Can you work these out from the model? Positions are in its coordinate system, mm. A direction names the side the tool comes from. Round coordinates to 2 decimals unless told otherwise and drop trailing zeros. Loops run counter-clockwise (first coordinate to the right, second up) from the corner with the lowest first, then second, coordinate; pieces in that order, holes last.
from build123d import *

# Parameters (mm, degrees)
SKETCH1_W           = 80
SKETCH1_H           = 160
SKETCH1_R           = 1.25
SKETCH1_R_2         = 1.5
SKETCH1_R_3         = 3.175
SKETCH1_W_2         = 25
SKETCH1_H_2         = 10
BOSS_EXTRUDE1_DEPTH = 3
SKETCH2_W           = 5
SKETCH2_H           = 25
BOSS_EXTRUDE2_DEPTH = 14
FILLET1_R           = 1
FILLET2_R           = 3
FILLET3_R           = 3
SKETCH4_R           = 1.25
CUT_EXTRUDE1_DEPTH  = 180.691402132
SKETCH6_R           = 2
CUT_EXTRUDE2_DEPTH  = 8.89
LPATTERN1_COUNT     = 6
LPATTERN1_PITCH     = 10
FILLET4_R           = 2


with BuildPart() as part:
    # Sketch1 → Boss-Extrude1 (new body)
    with BuildSketch(Plane(origin=(0, 0, 0), x_dir=(1, 0, 0), z_dir=(0, 1, 0))):
        with Locations((40, 80)):
            Rectangle(SKETCH1_W, SKETCH1_H)
        with Locations(Location((8, 130, 0), (0, 0, 270))):
            Circle(SKETCH1_R, mode=Mode.SUBTRACT)
        with Locations(Location((16, 130, 0), (0, 0, 270))):
            Circle(SKETCH1_R, mode=Mode.SUBTRACT)
        with Locations(Location((24, 130, 0), (0, 0, 270))):
            Circle(SKETCH1_R, mode=Mode.SUBTRACT)
        with Locations(Location((24, 122, 0), (0, 0, 270))):
            Circle(SKETCH1_R, mode=Mode.SUBTRACT)
        with Locations(Location((24, 114, 0), (0, 0, 270))):
            Circle(SKETCH1_R, mode=Mode.SUBTRACT)
        with Locations(Location((16, 114, 0), (0, 0, 270))):
            Circle(SKETCH1_R, mode=Mode.SUBTRACT)
        with Locations(Location((8, 114, 0), (0, 0, 270))):
            Circle(SKETCH1_R, mode=Mode.SUBTRACT)
        with Locations(Location((8, 122, 0), (0, 0, 270))):
            Circle(SKETCH1_R, mode=Mode.SUBTRACT)
        with Locations(Location((72, 130, 0), (0, 0, 90))):
            Circle(SKETCH1_R, mode=Mode.SUBTRACT)
        with Locations(Location((72, 122, 0), (0, 0, 90))):
            Circle(SKETCH1_R, mode=Mode.SUBTRACT)
        with Locations(Location((72, 114, 0), (0, 0, 90))):
            Circle(SKETCH1_R, mode=Mode.SUBTRACT)
        with Locations(Location((64, 114, 0), (0, 0, 90))):
            Circle(SKETCH1_R, mode=Mode.SUBTRACT)
        with Locations(Location((64, 130, 0), (0, 0, 90))):
            Circle(SKETCH1_R, mode=Mode.SUBTRACT)
        with Locations(Location((56, 130, 0), (0, 0, 90))):
            Circle(SKETCH1_R, mode=Mode.SUBTRACT)
        with Locations(Location((56, 122, 0), (0, 0, 90))):
            Circle(SKETCH1_R, mode=Mode.SUBTRACT)
        with Locations(Location((56, 114, 0), (0, 0, 90))):
            Circle(SKETCH1_R, mode=Mode.SUBTRACT)
        with Locations(Location((40, 17, 0), (0, 0, 270))):
            Circle(SKETCH1_R_2, mode=Mode.SUBTRACT)
        with Locations(Location((40, 74.5, 0), (0, 0, 270))):
            Circle(SKETCH1_R_2, mode=Mode.SUBTRACT)
        with Locations(Location((7, 7, 0), (0, 0, 270))):
            Circle(SKETCH1_R_3, mode=Mode.SUBTRACT)
        with Locations(Location((73, 7, 0), (0, 0, 90))):
            Circle(SKETCH1_R_3, mode=Mode.SUBTRACT)
        with Locations((40, 100)):
            Rectangle(SKETCH1_W_2, SKETCH1_H_2, mode=Mode.SUBTRACT)
    extrude(amount=BOSS_EXTRUDE1_DEPTH)

    # Sketch2 → Boss-Extrude2 (add)
    with BuildSketch(Plane(origin=(0, 3, 0), x_dir=(1, 0, 0), z_dir=(0, 1, 0))):
        with Locations((2.5, 27.5)):
            Rectangle(SKETCH2_W, SKETCH2_H)
        with Locations((77.5, 27.5)):
            Rectangle(SKETCH2_W, SKETCH2_H)
    extrude(amount=BOSS_EXTRUDE2_DEPTH)

    # Fillet1
    fillet1_edges = [part.edges().sort_by_distance(p)[0] for p in [
        (77.5, 3, -15),
        (75, 3, -27.5),
        (77.5, 3, -40),
        (2.5, 3, -40),
        (5, 3, -27.5),
        (2.5, 3, -15),
    ]]
    fillet(fillet1_edges, radius=FILLET1_R)

    # Fillet2
    fillet2_edges = [part.edges().sort_by_distance(p)[0] for p in [
        (0, 1.5, -160),
        (80, 1.5, -160),
        (80, 1.5, 0),
        (0, 1.5, 0),
    ]]
    fillet(fillet2_edges, radius=FILLET2_R)

    # Fillet3
    fillet3_edges = [part.edges().sort_by_distance(p)[0] for p in [
        (77.5, 17, -40),
        (77.5, 17, -15),
        (2.5, 17, -15),
        (2.5, 17, -40),
    ]]
    fillet(fillet3_edges, radius=FILLET3_R)

    # Sketch4 → Cut-Extrude1 (cut, through all)
    with BuildSketch(Plane.ZY):
        with Locations((-27.5, 8)):
            Circle(SKETCH4_R)
        with Locations((-35.5, 13)):
            Circle(SKETCH4_R)
        with Locations(Location((-19.5, 13, 0), (0, 0, 180))):
            Circle(SKETCH4_R)
    extrude(amount=-CUT_EXTRUDE1_DEPTH, mode=Mode.SUBTRACT)

    # Sketch6 → Cut-Extrude2 (cut)
    with BuildSketch(Plane(origin=(0, 3, 0), x_dir=(1, 0, 0), z_dir=(0, 1, 0))):
        with Locations(Location((6, 99.467444438, 0), (0, 0, 270))):
            Circle(SKETCH6_R)
        with Locations(Location((74, 99.467444438, 0), (0, 0, 270))):
            Circle(SKETCH6_R)
    cut_extrude2 = extrude(amount=-CUT_EXTRUDE2_DEPTH, mode=Mode.SUBTRACT)

    # LPattern1: Cut-Extrude2 ×6
    with Locations(*[(0, 0, i * LPATTERN1_PITCH) for i in range(1, LPATTERN1_COUNT)]):
        add(cut_extrude2, mode=Mode.SUBTRACT)

    # Fillet4
    fillet4_edges = [part.edges().sort_by_distance(p)[0] for p in [
        (52.5, 1.5, -95),
        (52.5, 1.5, -105),
        (27.5, 1.5, -105),
        (27.5, 1.5, -95),
    ]]
    fillet(fillet4_edges, radius=FILLET4_R)


solid = part.part
(1) If we mould it in two halves opening along Z, with no side actions, what happens to faces 4 (the flat face through (0, 2.8, -56.8)), 5 (the cylindrical face through (75.983, 1.521, -99.728)), 6 (the cylindrical face through (6.088, 1.521, -91.466)), 7 (the cylindrical face through (79.1, 1.52, -159.14))? For each: released by +Z, released by -Z, zero draft, split by the parting line, or undercut.
Worked answers:
face 4: zero draft
face 5: undercut
face 6: undercut
face 7: released by -Z
(2) If we section it at B-B, the plane x = 40: List the corners of the cut face in (y, z) for me, then the cut area to 3 significant figures.
Worked answers:
outline: (0, -160) - (3, -160) - (3, -105) - (0, -105) - close; (0, -95) - (3, -95) - (3, -76) - (0, -76) - close; (0, -73) - (3, -73) - (3, -18.5) - (0, -18.5) - close; (0, -15.5) - (3, -15.5) - (3, 0) - (0, 0) - close
area: 432 mm2
(3) If I drill on line 1 (Z direction, x = 64, y = 2.1); line 2 (Z direction, x = 76, y = 7.75); line 3 (X direction, y = 2.75, z = -8), over which ranges is the centre line in solid material (lowest first)?
Worked answers:
line 1: z = -160 to -131.25, -128.75 to -115.25, -112.75 to 0
line 2: z = -40 to -28.72, -26.28 to -15
line 3: x = 0 to 3.99, 10.01 to 69.99, 76.01 to 80
(4) If we section it at C-C, the plane z = -111: List the corners of the cut face in (x, y) for me.
Worked answers:
outline: (0, 0) - (80, 0) - (80, 3) - (0, 3) - close
(5) If we section it at A-A, the plane z = -7: List the corners of the cut face in (x, y) for me (3 decimals).
Worked answers:
outline: (0, 0) - (3.825, 0) - (3.825, 3) - (0, 3) - close; (10.175, 0) - (69.825, 0) - (69.825, 3) - (10.175, 3) - close; (76.175, 0) - (80, 0) - (80, 3) - (76.175, 3) - close
(6) For faces 1 (the flat face through (40, 1, -95)), 2 (the cylindrical face through (77.54, 16.1, -15.86)), 3 (the flat face through (5, 10, -27)), which set-ups out of +Z, -Z, +X, -X, +Y, -Y let a thin tool reach every point of the face, with its end or its side?
Worked answers:
face 1: +Y, -Y
face 2: +Z, +X, -X, +Y
face 3: +Z, -Z, +Y
(7) Will these pins go through, and if not, where does the flat tip stop? P1, Ø3, axis at x = 56, z = -122, coming from the -Y side; P2, Ø3, axis at x = 8, z = -122, coming from the +Y side; P3, Ø2.5, axis at x = 3, y = 7, coming from the -Z side.
Worked answers:
P1: stops at y = 0
P2: stops at y = 3
P3: stops at z = -40
